The model under review builds one solid part; all positions refer to its coordinate system, in mm. Give positions to 0.01 mm unless a question says otherwise; leave off trailing zeros. Loops run counter-clockwise (first coordinate to the right, second up) from the corner with the lowest first, then second, coordinate; pieces in that order, holes last. Notation, with made-up numbers: M 76.5,38 L 86.5,38 A20 ccw 86.5,63 Z; hole C 59.5,-3 d2. An arc over 180 degrees is marked long. One line per item, written item: value. Start each with the question number.
Q1. For pin 1 (1.5 mm diameter, centred on y = 10.5, z = 1, fed in from -X); pin 2 (1.5 mm diameter, centred on x = 48.5, z = 0.5, fed in from -Y) (3 decimals), all flat-tipped, find the tip position at first contact; note any pin that passes through.
Q2. Mouldability with a two-part tool opening along X and no side actions: class faces 1 (the face through (39, 16, 3.175)), 2 (the face through (3, 16, 2)), 3 (the face through (75.19, 12.56, 1.57)), 4 (the face through (12.35, 17.99, 1.57)) as released by +X, released by -X, zero draft, split by the parting line, or undercut.
Q3. We need section D-D on y = 6.25. Write out the cut boundary in (x, z) (3 decimals), plus the area to 3 significant figures.
Q4. We need section C-C on x = 12. Write out the cut boundary in (y, z) (1 decimal), plus the area to 3 significant figures.
Q5. We need section B-B on x = 28.75. Write out the cut boundary in (y, z) (3 decimals).
Q6. To check wall thickness, follow line 1 along Y through (x, z) = (19, 0.9); line 2 along Y through (x, z) = (28.75, 2.2); line 3 along X through (y, z) = (16.5, 1.45). State the ranges of each line that lie inside material, in increasing order. Write a range as from..to.
Q7. We need section A-A on y = 16. Write out the cut boundary in (x, z) (3 decimals).
```python
from build123d import *

# Parameters (mm, degrees)
SKETCH1_R           = 1.1
SKETCH1_R_2         = 5
BOSS_EXTRUDE1_DEPTH = 3.175
CUT_EXTRUDE1_DEPTH  = 3.175
FILLET1_R           = 4


with BuildPart() as part:
    # Sketch1 → Boss-Extrude1 (new body)
    with BuildSketch(Plane.XY):
        with BuildLine():
            Line((19, 0), (76, 0))
            Line((76, 0), (76, 32))
            Line((76, 32), (19, 32))
            ThreePointArc((19, 32), (3, 16), (19, 0))
        make_face()
        with Locations((25.894291117, 22.894291117)):
            Circle(SKETCH1_R, mode=Mode.SUBTRACT)
        with Locations((19, 25.75)):
            Circle(SKETCH1_R, mode=Mode.SUBTRACT)
        with Locations((28.75, 16)):
            Circle(SKETCH1_R, mode=Mode.SUBTRACT)
        with Locations((25.894291117, 9.105708883)):
            Circle(SKETCH1_R, mode=Mode.SUBTRACT)
        with Locations((19, 6.25)):
            Circle(SKETCH1_R, mode=Mode.SUBTRACT)
        with Locations((12.105708883, 9.105708883)):
            Circle(SKETCH1_R, mode=Mode.SUBTRACT)
        with Locations((9.25, 16)):
            Circle(SKETCH1_R, mode=Mode.SUBTRACT)
        with Locations((12.105708883, 22.894291117)):
            Circle(SKETCH1_R, mode=Mode.SUBTRACT)
        with Locations((19, 16)):
            Circle(SKETCH1_R_2, mode=Mode.SUBTRACT)
        with Locations((26.160066377, 18.965796601)):
            Circle(SKETCH1_R, mode=Mode.SUBTRACT)
        with Locations((21.965796601, 23.160066377)):
            Circle(SKETCH1_R, mode=Mode.SUBTRACT)
        with Locations((26.160066377, 13.034203399)):
            Circle(SKETCH1_R, mode=Mode.SUBTRACT)
        with Locations((21.965796601, 8.839933623)):
            Circle(SKETCH1_R, mode=Mode.SUBTRACT)
        with Locations((16.034203399, 8.839933623)):
            Circle(SKETCH1_R, mode=Mode.SUBTRACT)
        with Locations((11.839933623, 13.034203399)):
            Circle(SKETCH1_R, mode=Mode.SUBTRACT)
        with Locations((11.839933623, 18.965796601)):
            Circle(SKETCH1_R, mode=Mode.SUBTRACT)
        with Locations((16.034203399, 23.160066377)):
            Circle(SKETCH1_R, mode=Mode.SUBTRACT)
    extrude(amount=BOSS_EXTRUDE1_DEPTH)

    # Sketch2 → Cut-Extrude1 (cut)
    with BuildSketch(Plane.XY.offset(3.175)):
        Polygon((76, 32), (76, 20), (36, 32), align=None)
        Polygon((76, 0), (76, 12), (36, 0), align=None)
    extrude(amount=-CUT_EXTRUDE1_DEPTH, mode=Mode.SUBTRACT)

    # Fillet1
    fillet1_edges = [part.edges().sort_by_distance(p)[0] for p in [
        (36, 0, 1.5875),
        (76, 12, 1.5875),
        (36, 32, 1.5875),
        (76, 20, 1.5875),
    ]]
    fillet(fillet1_edges, radius=FILLET1_R)


solid = part.part
```
Solved:
1. pin 1: x = 3.72
1. pin 2: y = 3.525
2. face 1: zero draft
2. face 2: released by -X
2. face 3: released by +X
2. face 4: undercut
3. outline: M 6.314,0 L 17.9,0 L 17.9,3.175 L 6.314,3.175 Z; M 20.1,0 L 56.833,0 L 56.833,3.175 L 20.1,3.175 Z
3. area: 153 mm2
4. outline: M 1.6,0 L 8,0 L 8,3.2 L 1.6,3.2 Z; M 10.2,0 L 11.9,0 L 11.9,3.2 L 10.2,3.2 Z; M 14.1,0 L 17.9,0 L 17.9,3.2 L 14.1,3.2 Z; M 20.1,0 L 21.8,0 L 21.8,3.2 L 20.1,3.2 Z; M 24,0 L 30.4,0 L 30.4,3.2 L 24,3.2 Z
4. area: 63.6 mm2
5. outline: M 0,0 L 14.9,0 L 14.9,3.175 L 0,3.175 Z; M 17.1,0 L 32,0 L 32,3.175 L 17.1,3.175 Z
6. line 1: 0..5.15, 7.35..11, 21..24.65, 26.85..32
6. line 2: 0..14.9, 17.1..32
6. line 3: 3.01..8.27, 10.23..14.03, 23.97..27.77, 29.73..76
7. outline: M 3,0 L 8.15,0 L 8.15,3.175 L 3,3.175 Z; M 10.35,0 L 14,0 L 14,3.175 L 10.35,3.175 Z; M 24,0 L 27.65,0 L 27.65,3.175 L 24,3.175 Z; M 29.85,0 L 76,0 L 76,3.175 L 29.85,3.175 Z
